Check sheet for the modelled part. Datum: model origin and axes. Units: mm. A direction names the side the tool comes from. Give positions to 0.01 mm unless a question says otherwise; leave off trailing zeros. Write each loop counter-clockwise with the first axis right and the second up, starting at its lowest first coordinate (ties: lowest second). Pieces come first, ordered by that corner, then holes.
from build123d import *

# Parameters (mm, degrees)
EXTRUDE_1_DEPTH     = 8
CUT_EXTRUDE_1_DEPTH = 9
SKETCH_3_R          = 1.65
CUT_EXTRUDE_2_DEPTH = 26
SKETCH_4_R          = 3
CUT_EXTRUDE_3_DEPTH = 3.3
CUT_EXTRUDE_4_DEPTH = 3


with BuildPart() as part:
    # 草图1 → 凸台-拉伸1 (new body)
    with BuildSketch(Plane.XY):
        Polygon((-10, 25), (10, 25), (10, 10), (15, 10), (15, 0), (-15, 0), (-15, 10), (-10, 10), align=None)
    extrude(amount=EXTRUDE_1_DEPTH)

    # 草图2 → 切除-拉伸1 (cut, through all)
    with BuildSketch(Plane.XY.offset(8)):
        with BuildLine():
            Line((-1, 25), (1, 25))
            Line((1, 25), (1, 14.872983346))
            ThreePointArc((1, 14.872983346), (0, 7), (-1, 14.872983346))
            Line((-1, 14.872983346), (-1, 25))
        make_face()
    extrude(amount=-CUT_EXTRUDE_1_DEPTH, mode=Mode.SUBTRACT)

    # 草图3 → 切除-拉伸2 (cut, through all)
    with BuildSketch(Plane.ZY.offset(10)):
        with Locations((4, 20)):
            Circle(SKETCH_3_R)
    extrude(amount=-CUT_EXTRUDE_2_DEPTH, mode=Mode.SUBTRACT)

    # 草图4 → 切除-拉伸3 (cut)
    with BuildSketch(Plane.ZY.offset(10)):
        with Locations((4, 20)):
            Circle(SKETCH_4_R)
    extrude(amount=-CUT_EXTRUDE_3_DEPTH, mode=Mode.SUBTRACT)

    # 草图5 → 切除-拉伸4 (cut)
    with BuildSketch(Plane(origin=(10, 0, 0), x_dir=(0, 0, -1), z_dir=(1, 0, 0))):
        Polygon((-7.348631561, 20), (-5.674315781, 17.1), (-2.325684219, 17.1), (-0.651368439, 20), (-2.325684219, 22.9), (-5.674315781, 22.9), align=None)
    extrude(amount=-CUT_EXTRUDE_4_DEPTH, mode=Mode.SUBTRACT)


solid = part.part
1) Gauge pin test, flat ends, axial feed: pin 1 (3 mm diameter, centred on x = -0.5, y = 16.5, fed in from +Z); pin 2 (4 mm diameter, centred on y = 21.5, z = 4.5, fed in from -X); pin 3 (2.5 mm diameter, centred on x = 11.5, z = 3.5, fed in from +Y); pin 4 (1.5 mm diameter, centred on y = 14.5, z = 4, fed in from +X). Record the tip position at first contact, or that the pin passes through.
2) Sectioned sample at B-B on z = 4. Record the boundary of the cut face in (x, y), then the cut area to 3 significant figures.
3) Sectioned sample at C-C on x = 0. Record the boundary of the cut face in (y, z), then the cut area to 3 significant figures.
4) Scan lines: L1, parallel to X at y = 18, z = 3.75; L2, parallel to Y at x = 2.55, z = 4; L3, parallel to Y at x = 8, z = 3.5. Record each from-to range of solid material in increasing order.
5) Sectioned sample at D-D on z = 1.5. Record the boundary of the cut face in (x, y), then the cut area to 3 significant figures.
6) Sectioned sample at A-A on y = 11. Record the boundary of the cut face in (x, z), then the cut area to 3 significant figures.
7) Draft check along Y on faces 1 (the flat face through (-3, 7, 8)), 2 (the flat face through (12, 10, 4)), 3 (the flat face through (-6.7, 18.7, 5.3)). Enter one of: +Y half, -Y half, draft (parallel to the pull), parting line (faces both ways), or undercut.
8) Access from +Z, -Z, +X, -X, +Y, -Y to the whole of each face (thin tool, end or side, straight path). Record for faces 4 (the cylindrical face through (3.958, 21.636, 3.785)), 5 (the flat face through (-13, 10, 4)), 6 (the flat face through (-6, 25, 4)), 7 (the flat face through (7, 21.3, 2.6)), 8 (the flat face through (10, 16, 4)).
Answers below:
1. pin 1: stops at z = 8
1. pin 2: stops at x = -10
1. pin 3: stops at y = 10
1. pin 4: stops at x = 10
2. outline: (-15, 0) - (15, 0) - (15, 10) - (10, 10) - (10, 17.1) - (7, 17.1) - (7, 18.35) - (1, 18.35) - (1, 14.87) arc R4 cw (long way) to (-1, 14.87) - (-1, 18.35) - (-6.7, 18.35) - (-6.7, 17) - (-10, 17) - (-10, 10) - (-15, 10) - close; (-10, 23) - (-6.7, 23) - (-6.7, 21.65) - (-1, 21.65) - (-1, 25) - (-10, 25) - close; (1, 21.65) - (7, 21.65) - (7, 22.9) - (10, 22.9) - (10, 25) - (1, 25) - close
2. area: 454 mm2
3. outline: (0, 0) - (7, 0) - (7, 8) - (0, 8) - close
3. area: 56.0 mm2
4. L1: x = -6.7 to -1, 1 to 7
4. L2: y = 0 to 7.92, 14.08 to 18.35, 21.65 to 25
4. L3: y = 0 to 17.1, 22.9 to 25
5. outline: (-15, 0) - (15, 0) - (15, 10) - (10, 10) - (10, 18.53) - (7, 18.53) - (7, 21.47) - (10, 21.47) - (10, 25) - (1, 25) - (1, 14.87) arc R4 cw (long way) to (-1, 14.87) - (-1, 25) - (-10, 25) - (-10, 21.66) - (-6.7, 21.66) - (-6.7, 18.34) - (-10, 18.34) - (-10, 10) - (-15, 10) - close
5. area: 510 mm2
6. outline: (-10, 0) - (-4, 0) - (-4, 8) - (-10, 8) - close; (4, 0) - (10, 0) - (10, 8) - (4, 8) - close
6. area: 96.0 mm2
7. face 1: draft
7. face 2: +Y half
7. face 3: undercut
8. face 4: +X, -X
8. face 5: +Z, -Z, -X, +Y
8. face 6: +Z, -Z, +X, -X, +Y
8. face 7: +X
8. face 8: +Z, -Z, +X, +Y
